from build123d import *

# Parameters (mm, degrees)
F0_R     = 3.175
F1_DEPTH = 6.35


with BuildPart() as f1:
    # F0 (on Front) → F1 (new body)
    with BuildSketch(Plane.XZ):
        with Locations((0.01724, -0.018653)):
            Circle(F0_R)
        with BuildLine():
            ThreePointArc((1.778428, 0.007274), (1.778439, 0.00365), (1.778443, 2.5e-05))
            Line((1.778443, 2.5e-05), (2.05225, -0.145481))
            ThreePointArc((2.05225, -0.145481), (2.042521, -0.246727), (2.027738, -0.347359))
            Line((2.027738, -0.347359), (1.724364, -0.435232))
            ThreePointArc((1.724364, -0.435232), (1.723473, -0.438745), (1.722576, -0.442256))
            Line((1.722576, -0.442256), (1.951595, -0.651284))
            ThreePointArc((1.951595, -0.651284), (1.916993, -0.74693), (1.877648, -0.840723))
            Line((1.877648, -0.840723), (1.561952, -0.85039))
            ThreePointArc((1.561952, -0.85039), (1.560216, -0.853571), (1.558473, -0.856749))
            Line((1.558473, -0.856749), (1.728314, -1.116165))
            ThreePointArc((1.728314, -1.116165), (1.671013, -1.2002), (1.609579, -1.281263))
            Line((1.609579, -1.281263), (1.301397, -1.212115))
            ThreePointArc((1.301397, -1.212115), (1.298924, -1.214765), (1.296446, -1.217409))
            Line((1.296446, -1.217409), (1.396437, -1.510913))
            ThreePointArc((1.396437, -1.510913), (1.320038, -1.578058), (1.240374, -1.641295))
            Line((1.240374, -1.641295), (0.959071, -1.497679))
            ThreePointArc((0.959071, -1.497679), (0.956017, -1.49963), (0.952959, -1.501575))
            Line((0.952959, -1.501575), (0.976817, -1.810725))
            ThreePointArc((0.976817, -1.810725), (0.886119, -1.85676), (0.793232, -1.8982))
            Line((0.793232, -1.8982), (0.556482, -1.689137))
            ThreePointArc((0.556482, -1.689137), (0.553039, -1.690268), (0.549593, -1.691391))
            Line((0.549593, -1.691391), (0.495819, -1.996762))
            ThreePointArc((0.495819, -1.996762), (0.396523, -2.018795), (0.296248, -2.035833))
            Line((0.296248, -2.035833), (0.118928, -1.774462))
            ThreePointArc((0.118928, -1.774462), (0.115311, -1.7747), (0.111695, -1.774932))
            Line((0.111695, -1.774932), (-0.016332, -2.057335))
            ThreePointArc((-0.016332, -2.057335), (-0.117989, -2.053982), (-0.21935, -2.045547))
            Line((-0.21935, -2.045547), (-0.326099, -1.74829))
            ThreePointArc((-0.326099, -1.74829), (-0.329661, -1.747622), (-0.333222, -1.746946))
            Line((-0.333222, -1.746946), (-0.527457, -1.988639))
            ThreePointArc((-0.527457, -1.988639), (-0.625087, -1.96011), (-0.721166, -1.926732))
            Line((-0.721166, -1.926732), (-0.750636, -1.612266))
            ThreePointArc((-0.750636, -1.612266), (-0.75392, -1.610733), (-0.757201, -1.609194))
            Line((-0.757201, -1.609194), (-1.005441, -1.794989))
            ThreePointArc((-1.005441, -1.794989), (-1.092908, -1.743077), (-1.177668, -1.686854))
            Line((-1.177668, -1.686854), (-1.128008, -1.374938))
            ThreePointArc((-1.128008, -1.374938), (-1.130808, -1.372637), (-1.133602, -1.37033))
            Line((-1.133602, -1.37033), (-1.420248, -1.488553))
            ThreePointArc((-1.420248, -1.488553), (-1.492058, -1.41652), (-1.560173, -1.340984))
            Line((-1.560173, -1.340984), (-1.434503, -1.051218))
            ThreePointArc((-1.434503, -1.051218), (-1.436642, -1.048293), (-1.438775, -1.045363))
            Line((-1.438775, -1.045363), (-1.745817, -1.088586))
            ThreePointArc((-1.745817, -1.088586), (-1.797456, -1.000958), (-1.844646, -0.910855))
            Line((-1.844646, -0.910855), (-1.650863, -0.661446))
            ThreePointArc((-1.650863, -0.661446), (-1.652207, -0.65808), (-1.653545, -0.654712))
            Line((-1.653545, -0.654712), (-1.961689, -0.620219))
            ThreePointArc((-1.961689, -0.620219), (-1.989914, -0.522501), (-2.013214, -0.423494))
            Line((-2.013214, -0.423494), (-1.763493, -0.230112))
            ThreePointArc((-1.763493, -0.230112), (-1.763958, -0.226518), (-1.764416, -0.222923))
            Line((-1.764416, -0.222923), (-2.054301, -0.112881))
            ThreePointArc((-2.054301, -0.112881), (-2.057338, -0.011215), (-2.055284, 0.090477))
            Line((-2.055284, 0.090477), (-1.765316, 0.21568))
            ThreePointArc((-1.765316, 0.21568), (-1.764873, 0.219277), (-1.764422, 0.222873))
            Line((-1.764422, 0.222873), (-2.017834, 0.401549))
            ThreePointArc((-2.017834, 0.401549), (-1.995492, 0.500777), (-1.968213, 0.598762))
            Line((-1.968213, 0.598762), (-1.656218, 0.64792))
            ThreePointArc((-1.656218, 0.64792), (-1.654894, 0.651294), (-1.653563, 0.654665))
            Line((-1.653563, 0.654665), (-1.854579, 0.890748))
            ThreePointArc((-1.854579, 0.890748), (-1.808262, 0.981303), (-1.757472, 1.069426))
            Line((-1.757472, 1.069426), (-1.443054, 1.039449))
            ThreePointArc((-1.443054, 1.039449), (-1.440932, 1.042388), (-1.438805, 1.045322))
            Line((-1.438805, 1.045322), (-1.574794, 1.323979))
            ThreePointArc((-1.574794, 1.323979), (-1.507412, 1.40017), (-1.436302, 1.472893))
            Line((-1.436302, 1.472893), (-1.139217, 1.365666))
            ThreePointArc((-1.139217, 1.365666), (-1.136432, 1.367984), (-1.133641, 1.370297))
            Line((-1.133641, 1.370297), (-1.196058, 1.674019))
            ThreePointArc((-1.196058, 1.674019), (-1.111846, 1.731059), (-1.024884, 1.783813))
            Line((-1.024884, 1.783813), (-0.763799, 1.606072))
            ThreePointArc((-0.763799, 1.606072), (-0.760525, 1.607626), (-0.757247, 1.609172))
            Line((-0.757247, 1.609172), (-0.74217, 1.918874))
            ThreePointArc((-0.74217, 1.918874), (-0.646418, 1.953179), (-0.549069, 1.98265))
            Line((-0.549069, 1.98265), (-0.340389, 1.745564))
            ThreePointArc((-0.340389, 1.745564), (-0.336831, 1.746254), (-0.333272, 1.746937))
            Line((-0.333272, 1.746937), (-0.241649, 2.043159))
            ThreePointArc((-0.241649, 2.043159), (-0.140374, 2.052574), (-0.038754, 2.056909))
            Line((-0.038754, 2.056909), (0.104409, 1.775375))
            ThreePointArc((0.104409, 1.775375), (0.108027, 1.775159), (0.111644, 1.774935))
            Line((0.111644, 1.774935), (0.274056, 2.039066))
            ThreePointArc((0.274056, 2.039066), (0.374491, 2.022998), (0.473996, 2.001926))
            Line((0.473996, 2.001926), (0.542647, 1.693633))
            ThreePointArc((0.542647, 1.693633), (0.546097, 1.692524), (0.549545, 1.691407))
            Line((0.549545, 1.691407), (0.772541, 1.90685))
            ThreePointArc((0.772541, 1.90685), (0.865825, 1.86631), (0.956963, 1.821153))
            Line((0.956963, 1.821153), (0.946788, 1.505474))
            ThreePointArc((0.946788, 1.505474), (0.949854, 1.503541), (0.952916, 1.501602))
            Line((0.952916, 1.501602), (1.222484, 1.654819))
            ThreePointArc((1.222484, 1.654819), (1.302756, 1.592355), (1.379801, 1.525952))
            Line((1.379801, 1.525952), (1.291439, 1.22272))
            ThreePointArc((1.291439, 1.22272), (1.293928, 1.220086), (1.296411, 1.217446))
            Line((1.296411, 1.217446), (1.595614, 1.298811))
            ThreePointArc((1.595614, 1.298811), (1.65783, 1.218346), (1.71594, 1.134868))
            Line((1.71594, 1.134868), (1.554944, 0.863138))
            ThreePointArc((1.554944, 0.863138), (1.5567, 0.859968), (1.558449, 0.856793))
            Line((1.558449, 0.856793), (1.868486, 0.861193))
            ThreePointArc((1.868486, 0.861193), (1.908736, 0.767784), (1.944261, 0.672477))
            Line((1.944261, 0.672477), (1.720746, 0.449322))
            ThreePointArc((1.720746, 0.449322), (1.721658, 0.445815), (1.722563, 0.442305))
            Line((1.722563, 0.442305), (2.023954, 0.369463))
            ThreePointArc((2.023954, 0.369463), (2.03971, 0.268979), (2.050417, 0.167832))
            Line((2.050417, 0.167832), (1.778428, 0.007274))
        make_face(mode=Mode.SUBTRACT)
    extrude(amount=F1_DEPTH)


solid = f1.part
Build history of the part. All positions in model axes, mm. Round coordinates to 2 decimals unless told otherwise and drop trailing zeros. Write each loop counter-clockwise with the first axis right and the second up, starting at its lowest first coordinate (ties: lowest second). Pieces come first, ordered by that corner, then holes. Notation, with made-up numbers: (43.25, 3) - (83.25, 3) arc R19 cw to (83.25, 25) - close; hole circle Ø1 at (53, 32.25). An arc over 180 degrees is marked (long way). Use CSV: the item, a comma, the result in double quotes.
(1) Band-saw the part on B-B (x = 2.75). Write the cut outline in (y, z), plus the area to 3 significant figures.
Response:
outline,"(-6.35, -1.64) - (0, -1.64) - (0, 1.6) - (-6.35, 1.6) - close"
area,"20.5 mm²"
(2) Band-saw the part on A-A (z = -2.5). Write the cut outline in (x, y), plus the area to 3 significant figures.
Response:
outline,"(-1.96, -6.35) - (2, -6.35) - (2, 0) - (-1.96, 0) - close"
area,"25.2 mm²"
(3) Wall check: line 1 (X direction, y = -3, z = -1); line 2 (X direction, y = -1.75, z = -0.5); line 3 (Z direction, x = -1.25, y = -2). Give the ranges that are in metal, low to high.
Response:
line 1,"-3 to -1.8, 1.65 to 3.04"
line 2,"-3.12 to -2, 1.79 to 3.16"
line 3,"-2.93 to -1.42, 1.41 to 2.89"
(4) Pin check, flat tips, straight feed: P1, Ø1, axis at x = 0.5, z = 0, coming from the -Y side; P2, Ø1.5, axis at x = 2, z = -0.5, coming from the +Y side; P3, Ø1.5, axis at x = 2, y = -4, coming from the +Z side. Stop position of each tip, or through.
Response:
P1,"through"
P2,"y = 0"
P3,"z = 2.91"
